```python
from build123d import *

# Parameters (mm, degrees)
SKETCH_R     = 6.5
PAD_DEPTH    = 91
SKETCH001_R  = 4
PAD001_DEPTH = 10
SKETCH002_R  = 4
PAD002_DEPTH = 10


with BuildPart() as part:
    # Sketch → Pad (new body, symmetric)
    with BuildSketch(Plane.YZ):
        Circle(SKETCH_R)
    extrude(amount=PAD_DEPTH, both=True)

    # Sketch001 (on Face3 of Pad) → Pad001 (join)
    with BuildSketch(Plane.YZ.offset(91)):
        Circle(SKETCH001_R)
    extrude(amount=PAD001_DEPTH)

    # Sketch002 (on Face2 of Pad001) → Pad002 (join)
    with BuildSketch(Plane(origin=(-91, 0, 0), x_dir=(0, 1, 0), z_dir=(-1, 0, 0))):
        Circle(SKETCH002_R)
    extrude(amount=PAD002_DEPTH)


solid = part.part
```
CAD build for the part. Positions are in the model's coordinates, mm. A direction names the side the tool comes from. Round coordinates to 2 decimals unless told otherwise and drop trailing zeros. Write each loop counter-clockwise with the first axis right and the second up, starting at its lowest first coordinate (ties: lowest second). Pieces come first, ordered by that corner, then holes. Notation, with made-up numbers: (35, 54) - (56, 54) arc R18 cw to (56, 89) - close; hole circle Ø9 at (47, 44.25). An arc over 180 degrees is marked (long way). Return JSON: item names as keys, results as strings. Group by question number.
Item 1: 3-axis set-ups, long thin cutter, end or side, ignore diameter. For faces 1 (the face through (95.93, -0.867, -3.905)), 2 (the face through (-91, 3, 3)), 3 (the face through (1.274, -5.158, -3.955)): which of +Z, -Z, +X, -X, +Y, -Y reach the whole face in a straight line?
Item 2: Probe probe 1 along Z at (x, y) = (-7, -0.5); probe 2 along X at (y, z) = (-1, -5); probe 3 along Z at (x, y) = (41.5, 4.25). List the from-to ranges inside material, lowest first.
Item 3: Band-saw the part on A-A on z = 0. List the corners of the cut face in (x, y).
Item 4: Band-saw the part on C-C on x = 78.5. List the corners of the cut face in (y, z).
Item 5: Flat gauge pins, fed straight in: pin 1 Ø2 at (x, z) = (69.5, -4) entering from +Y; pin 2 Ø3 at (x, z) = (-67, -5) entering from -Y; pin 3 Ø1.5 at (x, y) = (46.5, 1) entering from -Z. Where does each tip first touch, or does it go through?
Resolved:
{
 "1": {"face 1": "+X", "face 2": "-X", "face 3": "+X, -X"},
 "2": {"probe 1": "z = -6.48 to 6.48", "probe 2": "x = -91 to 91", "probe 3": "z = -4.92 to 4.92"},
 "3": {"outline": "(-101, -4) - (-91, -4) - (-91, -6.5) - (91, -6.5) - (91, -4) - (101, -4) - (101, 4) - (91, 4) - (91, 6.5) - (-91, 6.5) - (-91, 4) - (-101, 4) - close"},
 "4": {"outline": "circle Ø13 at (0, 0)"},
 "5": {"pin 1": "stops at y = 5.77", "pin 2": "stops at y = -5.48", "pin 3": "stops at z = -6.5"}
}
